The listing builds one solid part. Answer for the finished solid, in the listing's coordinates (mm). Coordinates: 2 decimals unless noted, no trailing zeros. Order: outer loops, then holes, each group sorted by start corner. A loop starts at its lowest first (then second) coordinate and runs counter-clockwise, first axis right, second up. Notation, with made-up numbers: M 70,45.25 L 99,45.25 A18 cw 99,63.25 Z; hole C 78,41.25 d10. An arc over 180 degrees is marked long. One line per item, written item: value. Start each with the question number.
Q1. Straight lines are drawn through the part: line 1 along X through (y, z) = (2.5, -6.35) (1 decimal); line 2 along X through (y, z) = (4.5, 7); line 3 along Z through (x, y) = (7.5, 3) (3 decimals). For each, find the intervals that lie inside material, in ascending order. Write a range as [from, to].
Q2. The part is cut by section D-D on x = 52. Give the vertices of the cut face in (y, z), then the cut area to 3 significant figures.
Q3. Each of these flat-tipped pins is pushed along its axis until it touches: pin 1 Ø1.9 at (x, y) = (90.5, 4) entering from -Z; pin 2 Ø1.9 at (y, z) = (4.5, -16) entering from +X; pin 3 Ø3.5 at (x, z) = (157.8, -6.35) entering from +Y; pin 4 Ø3 at (x, y) = (131.5, 1) entering from +Z. Where does it stop, or does it pass through?
Q4. The part is cut by section C-C on y = 3.75. Give the number of separate pieces and of enclosed holes in the cut face, then the cut area to 3 significant figures.
Q5. The part is cut by section B-B on z = -2.5. Give the vertices of the cut face in (x, y).
```python
from build123d import *

# Parameters (mm, degrees)
SKETCH1_R           = 1.905
BOSS_EXTRUDE1_DEPTH = 6.35


with BuildPart() as part:
    # Sketch1 → Boss-Extrude1 (new body)
    with BuildSketch(Plane(origin=(0, 0, 0), x_dir=(1, 0, 0), z_dir=(0, 1, 0))):
        with BuildLine():
            Line((88.9, -6.35), (152.4, -6.35))
            Line((152.4, -6.35), (152.4, -9.525))
            Line((152.4, -9.525), (165.1, -9.525))
            Line((165.1, -9.525), (165.1, -6.35))
            Line((165.1, -6.35), (165.1, 0))
            Line((165.1, 0), (165.1, 12.7))
            ThreePointArc((165.1, 12.7), (163.240128061, 17.190128061), (158.75, 19.05))
            Line((158.75, 19.05), (156.845, 19.05))
            ThreePointArc((156.845, 19.05), (152.354871939, 17.190128061), (150.495, 12.7))
            Line((150.495, 12.7), (150.495, 6.35))
            ThreePointArc((150.495, 6.35), (148.635128061, 1.859871939), (144.145, 0))
            Line((144.145, 0), (20.955, 0))
            ThreePointArc((20.955, 0), (16.464871939, 1.859871939), (14.605, 6.35))
            Line((14.605, 6.35), (14.605, 38.1))
            ThreePointArc((14.605, 38.1), (12.745128061, 42.590128061), (8.255, 44.45))
            Line((8.255, 44.45), (6.35, 44.45))
            ThreePointArc((6.35, 44.45), (1.859871939, 42.590128061), (0, 38.1))
            Line((0, 38.1), (0, 0))
            Line((0, 0), (0, -6.35))
            Line((0, -6.35), (0, -9.525))
            Line((0, -9.525), (12.7, -9.525))
            Line((12.7, -9.525), (12.7, -6.35))
            Line((12.7, -6.35), (76.2, -6.35))
            Line((76.2, -6.35), (76.2, -9.525))
            Line((76.2, -9.525), (88.9, -9.525))
            Line((88.9, -9.525), (88.9, -6.35))
        make_face()
        with Locations(Location((7.3025, 31.75, 0), (0, 0, 270))):
            Circle(SKETCH1_R, mode=Mode.SUBTRACT)
        with Locations(Location((7.3025, 6.35, 0), (0, 0, 270))):
            Circle(SKETCH1_R, mode=Mode.SUBTRACT)
        with Locations(Location((157.7975, 6.353059153, 0), (0, 0, 270))):
            Circle(SKETCH1_R, mode=Mode.SUBTRACT)
    extrude(amount=BOSS_EXTRUDE1_DEPTH)


solid = part.part
```
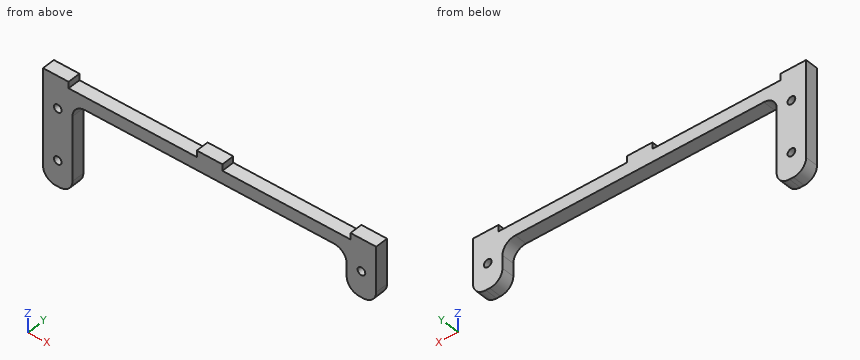
Output:
1. line 1: x = [0, 5.4], [9.2, 14.6], [150.5, 155.9], [159.7, 165.1]
1. line 2: x = [0, 12.7], [76.2, 88.9], [152.4, 165.1]
1. line 3: z = [-44.45, -33.645], [-29.855, -8.245], [-4.455, 9.525]
2. outline: M 0,0 L 6.35,0 L 6.35,6.35 L 0,6.35 Z
2. area: 40.3 mm^2
3. pin 1: stops at z = 0
3. pin 2: stops at x = 164.65
3. pin 3: passes through
3. pin 4: stops at z = 6.35
4. separate pieces: 1
4. enclosed holes: 3
4. area: 2,050 mm^2
5. outline: M 0,0 L 15.91,0 L 15.91,6.35 L 0,6.35 Z; M 149.19,0 L 165.1,0 L 165.1,6.35 L 149.19,6.35 Z
